Geometry: see drawing. Coordinates: mm, zero at the bounding-box minimum. Give positions to 0.01 mm unless a question says otherwise; leave off trailing zeros. Write each loop counter-clockwise with the first axis right and the second up, starting at its lowest first coordinate (ties: lowest second). Pieces come first, ordered by that corner, then holes. Notation, with made-up numbers: (77, -35.75) - (90, -35.75) arc R5 ccw to (90, -29.75) - close; hole circle Ø11 at (85.25, 35.25). An arc over 180 degrees is marked (long way). Use a Markdown table: item, result. Add a question column.
1. Section query C-C, the plane y = 70. Return loops of the section in (x, z), plus the area to 3 significant figures.
2. Material intervals for probe 1 along Y at (x, z) = (20, 1.75); probe 2 along X at (y, z) = (5, 3.3); probe 3 along Y at (x, z) = (19, 2.5), sorted ascending.
3. Section query A-A, the plane x = 10. Return loops of the section in (y, z).
4. Pin query (flat end, axial travel): pin 1 (1.3 mm diameter, centred on x = 20, y = 5, fed in from -Z); pin 2 (6.5 mm diameter, centred on x = 30, y = 70, fed in from +Z); pin 3 (2 mm diameter, centred on y = 19, z = 1.5, fed in from +X). Return the tip coordinate at first contact, or that it passes through.
5. Section query D-D, the plane z = 0.85. Return loops of the section in (x, y), plus the area to 3 significant figures.
6. Section query B-B, the plane y = 5. Return loops of the section in (x, z).
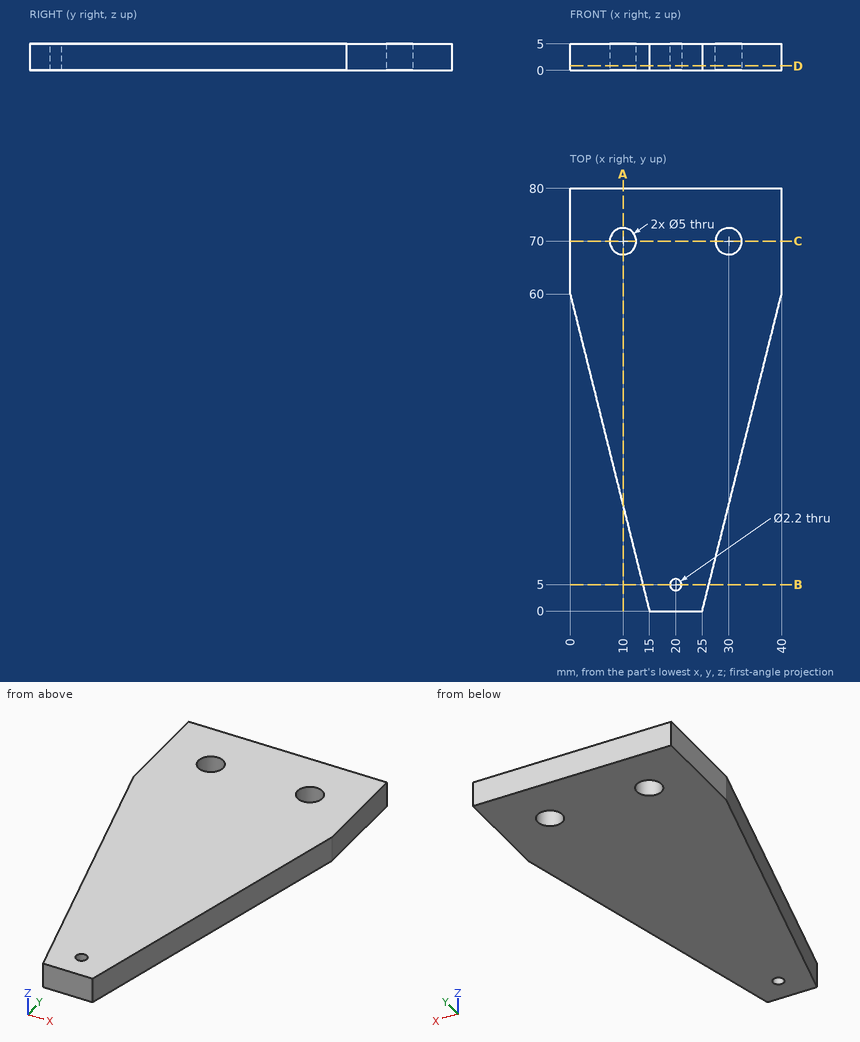
Result sheet:
| question | item | result |
|---|---|---|
| 1 | outline | (0, 0) - (7.5, 0) - (7.5, 5) - (0, 5) - close; (12.5, 0) - (27.5, 0) - (27.5, 5) - (12.5, 5) - close; (32.5, 0) - (40, 0) - (40, 5) - (32.5, 5) - close |
| 1 | area | 150 mm² |
| 2 | probe 1 | y = 0 to 3.9, 6.1 to 80 |
| 2 | probe 2 | x = 13.75 to 18.9, 21.1 to 26.25 |
| 2 | probe 3 | y = 0 to 4.54, 5.46 to 80 |
| 3 | outline | (20, 0) - (67.5, 0) - (67.5, 5) - (20, 5) - close; (72.5, 0) - (80, 0) - (80, 5) - (72.5, 5) - close |
| 4 | pin 1 | passes through |
| 4 | pin 2 | stops at z = 5 |
| 4 | pin 3 | stops at x = 30 |
| 5 | outline | (0, 60) - (15, 0) - (25, 0) - (40, 60) - (40, 80) - (0, 80) - close; hole circle Ø5 at (10, 70); hole circle Ø2.2 at (20, 5); hole circle Ø5 at (30, 70) |
| 5 | area | 2,260 mm² |
| 6 | outline | (13.75, 0) - (18.9, 0) - (18.9, 5) - (13.75, 5) - close; (21.1, 0) - (26.25, 0) - (26.25, 5) - (21.1, 5) - close |
